Check sheet for the modelled part. Datum: model origin and axes. Units: mm. A direction names the side the tool comes from. Round coordinates to 2 decimals unless told otherwise and drop trailing zeros. Order: outer loops, then holes, each group sorted by start corner. A loop starts at its lowest first (then second) coordinate and runs counter-clockwise, first axis right, second up. Notation, with made-up numbers: M -33,-4.5 L 2,-4.5 A30 ccw 2,18.5 Z; hole C 12.25,23.5 d6. An arc over 180 degrees is marked long. One line per item, written item: value. Start each with the question number.
(1) Cross-section at B-B, the plane x = 10. Enter the section's corners in (y, z), and give its area (3 significant figures).
(2) Access from +Z, -Z, +X, -X, +Y, -Y to the whole of each face (thin tool, end or side, straight path). Record for faces 4 (the face through (10, 20, 24)), 5 (the face through (10, 20, 0)).
(3) Cross-section at A-A, the plane z = 6. Enter the section's corners in (x, y).
(4) Cross-section at D-D, the plane x = 5.75. Enter the section's corners in (y, z).
(5) Release check for a two-part mould opening along Y. For faces 1 (the face through (10.14, 4.143, 31.301)), 2 (the face through (9.805, 17.934, 28.513)), 3 (the face through (10, 0, 20)) record: released by +Y, released by -Y, zero draft, split by the parting line, or undercut.
(6) Cross-section at C-C, the plane y = 30. Enter the section's corners in (x, z).
(7) Depth check by flat-ended pin: pin 1 Ø4.5 at (x, y) = (13.5, 30.5) entering from +Z; pin 2 Ø5 at (x, z) = (10, 30) entering from +Y. Enter the tip coordinate at first touch or a pass-through.
(8) Thickness scan on L1, parallel to Y at x = 10, z = 3.5; L2, parallel to Y at x = 8.5, z = 38.5; L3, parallel to Z at x = 8.5, y = 32. Record the ranges inside material, lowest first.
from build123d import *

# Parameters (mm, degrees)
SKETCH1_W                  = 20
SKETCH1_H                  = 20
BOSS_EXTRUDE1_DEPTH        = 40
SKETCH2_R                  = 6
CUT_EXTRUDE1_DEPTH         = 30
F_3_0MM_DOWEL_HOLE1_REACH  = 50.99
F_3_0MM_DOWEL_HOLE1_BORE_R = 1.5
SKETCH5_R                  = 2
CUT_EXTRUDE2_DEPTH         = 30
SKETCH6_W                  = 20
SKETCH6_H                  = 4
BOSS_EXTRUDE2_DEPTH        = 20
F_4_4_4_4_DIAMETER_HOLE1_D = 4.4
FILLET1_R                  = 5


with BuildPart() as part:
    # Sketch1 → Boss-Extrude1 (new body)
    with BuildSketch(Plane.XY):
        with Locations((10, 10)):
            Rectangle(SKETCH1_W, SKETCH1_H)
    extrude(amount=BOSS_EXTRUDE1_DEPTH)

    # Sketch2 → Cut-Extrude1 (cut)
    with BuildSketch(Plane(origin=(20, 0, 0), x_dir=(0, 0, -1), z_dir=(1, 0, 0))):
        with Locations((-30, 10)):
            Circle(SKETCH2_R)
    extrude(amount=-CUT_EXTRUDE1_DEPTH, mode=Mode.SUBTRACT)

    # Ø3.0mm Dowel Hole1 bore → Ø3.0mm Dowel Hole1 (cut, up to next)
    with BuildSketch(Plane(origin=(0, 20, 0), x_dir=(1, 0, 0), z_dir=(0, 1, 0)), mode=Mode.PRIVATE) as f_3_0mm_dowel_hole1_sk1:
        with Locations((10, -30)):
            Circle(F_3_0MM_DOWEL_HOLE1_BORE_R)
    f_3_0mm_dowel_hole1_tool1 = extrude(f_3_0mm_dowel_hole1_sk1.sketch, amount=-F_3_0MM_DOWEL_HOLE1_REACH, mode=Mode.PRIVATE) & part.part
    add(f_3_0mm_dowel_hole1_tool1.solids().sort_by_distance((10, 20, 30))[0], mode=Mode.SUBTRACT)

    # Sketch5 → Cut-Extrude2 (cut)
    with BuildSketch(Plane.ZY):
        with Locations((6, 10)):
            Circle(SKETCH5_R)
    extrude(amount=-CUT_EXTRUDE2_DEPTH, mode=Mode.SUBTRACT)

    # Sketch6 → Boss-Extrude2 (add)
    with BuildSketch(Plane(origin=(0, 20, 0), x_dir=(1, 0, 0), z_dir=(0, 1, 0))):
        with Locations((10, -2)):
            Rectangle(SKETCH6_W, SKETCH6_H)
    extrude(amount=BOSS_EXTRUDE2_DEPTH)

    # Ø4.4 (4.4) Diameter Hole1 (through all)
    with Locations(Plane.XY.offset(4)):
        with Locations((10, 30)):
            Hole(F_4_4_4_4_DIAMETER_HOLE1_D / 2)

    # Fillet1
    fillet1_edges = [part.edges().sort_by_distance(p)[0] for p in [
        (10, 20, 4),
    ]]
    fillet(fillet1_edges, radius=FILLET1_R)


solid = part.part
Values found:
1. outline: M 0,0 L 27.8,0 L 27.8,4 L 25,4 A5 cw 20,9 L 20,28.5 L 15.81,28.5 A6 cw long 15.81,31.5 L 20,31.5 L 20,40 L 0,40 Z; M 32.2,0 L 40,0 L 40,4 L 32.2,4 Z; hole C 10,6 d4
1. area: 730 mm^2
2. face 4: +Z, +X, -X, +Y
2. face 5: -Z, +X, -X, +Y, -Y
3. outline: M 0,0 L 20,0 L 20,8 L 0,8 Z; M 0,12 L 20,12 L 20,21 L 0,21 Z
4. outline: M 0,0 L 40,0 L 40,4 L 25,4 A5 cw 20,9 L 20,40 L 0,40 Z; hole C 10,30 d12; hole C 10,6 d4
5. face 1: undercut
5. face 2: zero draft
5. face 3: released by -Y
6. outline: M 0,0 L 7.8,0 L 7.8,4 L 0,4 Z; M 12.2,0 L 20,0 L 20,4 L 12.2,4 Z
7. pin 1: z = 4
7. pin 2: y = 20
8. L1: 0 to 27.8, 32.2 to 40
8. L2: 0 to 20
8. L3: 0 to 4
